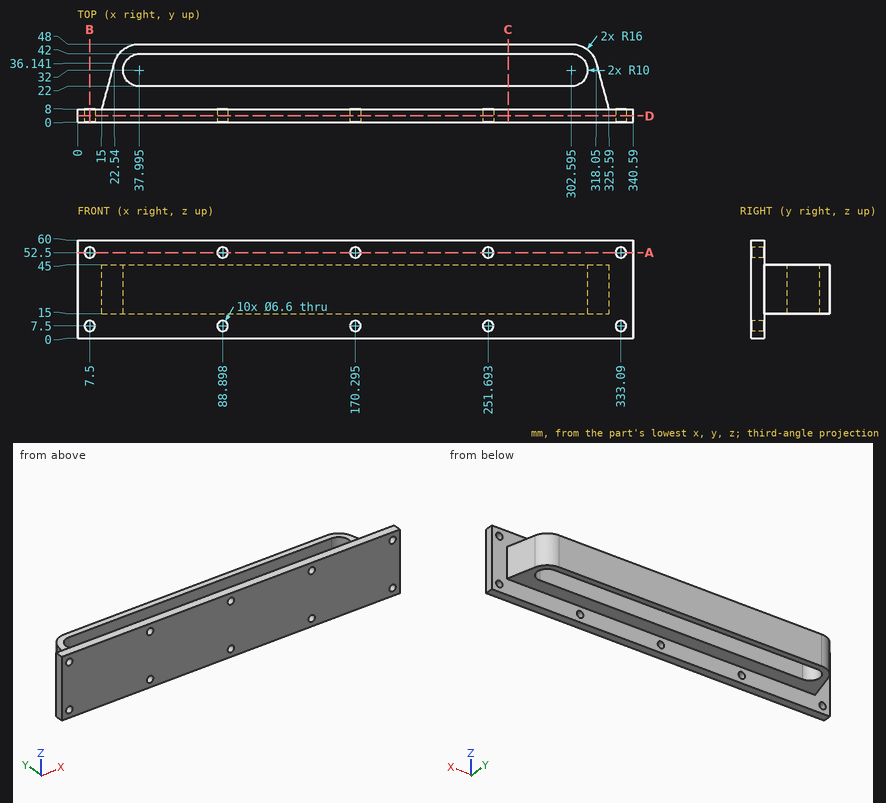
For this review, use the dimensioned drawing (mm, ordinates from the lowest corner) and the shaded views. Give positions to 0.01 mm unless a question says otherwise; leave off trailing zeros. Loops run counter-clockwise (first coordinate to the right, second up) from the corner with the lowest first, then second, coordinate; pieces in that order, holes last. Notation, with made-up numbers: (84.5, 67.5) -> (97.5, 67.5) arc R31 ccw to (97.5, 104.5) -> close; hole circle Ø5 at (-17.75, 37.5). An arc over 180 degrees is marked (long way). Use CSV: the item, a comma, the result in double quotes.
1. Consider section C-C, the plane x = 264. Write out the cut boundary in (y, z).
Result:
outline,"(0, 0) -> (8, 0) -> (8, 15) -> (22, 15) -> (22, 45) -> (8, 45) -> (8, 60) -> (0, 60) -> close; (42, 15) -> (48, 15) -> (48, 45) -> (42, 45) -> close"
2. For P1, Ø5, axis at y = 40.5, z = 39.5, coming from the +X side; P2, Ø5, axis at x = 114.5, y = 18, coming from the -Z side; P3, Ø4, axis at x = 7.5, z = 52.5, coming from the +Y side; P4, Ø7.5, axis at x = 7.5, z = 7.5, coming from the +Y side, all flat-tipped, find the tip position at first contact; note any pin that passes through.
Result:
P1,"stops at x = 317.43"
P2,"stops at z = 15"
P3,"passes through"
P4,"stops at y = 8"
3. Consider section B-B, the plane x = 7.5. Write out the cut boundary in (y, z).
Result:
outline,"(0, 0) -> (8, 0) -> (8, 4.2) -> (0, 4.2) -> close; (0, 10.8) -> (8, 10.8) -> (8, 49.2) -> (0, 49.2) -> close; (0, 55.8) -> (8, 55.8) -> (8, 60) -> (0, 60) -> close"
4. Consider section A-A, the plane z = 52.5. Write out the cut boundary in (x, y) (1 decimal), then the cut area to 3 significant figures.
Result:
outline,"(0, 0) -> (4.2, 0) -> (4.2, 8) -> (0, 8) -> close; (10.8, 0) -> (85.6, 0) -> (85.6, 8) -> (10.8, 8) -> close; (92.2, 0) -> (167, 0) -> (167, 8) -> (92.2, 8) -> close; (173.6, 0) -> (248.4, 0) -> (248.4, 8) -> (173.6, 8) -> close; (255, 0) -> (329.8, 0) -> (329.8, 8) -> (255, 8) -> close; (336.4, 0) -> (340.6, 0) -> (340.6, 8) -> (336.4, 8) -> close"
area,"2,460 mm²"
5. To check wall thickness, follow probe 1 along Z at (x, y) = (7, 5); probe 2 along X at (y, z) = (4.25, 52.5) (1 decimal); probe 3 along Y at (x, z) = (231, 22). State the ranges of each line that lie inside material, in increasing order. Write a range as from..to.
Result:
probe 1,"z = 0..4.24, 10.76..49.24, 55.76..60"
probe 2,"x = 0..4.2, 10.8..85.6, 92.2..167, 173.6..248.4, 255..329.8, 336.4..340.6"
probe 3,"y = 0..22, 42..48"
6. Consider section D-D, the plane y = 4. Count the separate pieces of the cut face and the enclosed holes in it, then the cut area to 3 significant figures.
Result:
separate pieces,"1"
enclosed holes,"10"
area,"20,100 mm²"
